from build123d import *

# Parameters (mm, degrees)
PAD018_DEPTH            = 12.35
PAD019_DEPTH            = 4.17
SKETCH036_R             = 1.5
POCKET011_DEPTH         = 5
FILLET014_R             = 0.3
BODY008_PLACEMENT_ANGLE = 180


with BuildPart() as part:
    # Sketch034 → Pad018 (new body)
    with BuildSketch(Plane.XY):
        Polygon((0, 23.8), (22.6, 23.8), (22.6, 19.97), (27.78, 19.97), (27.78, 17.33), (22.6, 17.33), (22.6, 0), (0, 0), (0, 17.33), (-5.18, 17.33), (-5.18, 19.97), (0, 19.97), align=None)
    extrude(amount=PAD018_DEPTH)

    # Sketch035 (on Face4 of Pad018) → Pad019 (join)
    with BuildSketch(Plane(origin=(0, 23.8, 0), x_dir=(-1, 0, 0), z_dir=(0, 1, 0))):
        with BuildLine():
            ThreePointArc((-10.895586, 8.809617), (-22.55, 6.175), (-10.895586, 3.540383))
            ThreePointArc((-10.895586, 3.540383), (-7.605, 6.175), (-10.895586, 8.809617))
        make_face()
    extrude(amount=PAD019_DEPTH)

    # Sketch036 (on Face10 of Pad019) → Pocket011 (cut)
    with BuildSketch(Plane(origin=(0, 19.97, 0), x_dir=(-1, 0, 0), z_dir=(0, 1, 0))):
        with Locations((-25.73, 6.175)):
            Circle(SKETCH036_R)
        with Locations((3.13, 6.175)):
            Circle(SKETCH036_R)
    extrude(amount=-POCKET011_DEPTH, mode=Mode.SUBTRACT)

    # Fillet014
    fillet014_edges = [part.edges().sort_by_distance(p)[0] for p in [
        (22.55, 27.97, 6.175),
        (7.605, 27.97, 6.175),
    ]]
    fillet(fillet014_edges, radius=FILLET014_R)


with BuildPart() as part_1:
    # Body008 placement: moved
    add(part.part.moved(Location((215.339996, 126.400008, -13.43))).rotate(Axis((215.339996, 126.400008, -13.43), (0, 1, 0)), BODY008_PLACEMENT_ANGLE))


solid = part_1.part
The model under review builds one solid part; all positions refer to its coordinate system, in mm. A direction names the side the tool comes from. Give positions to 0.01 mm unless a question says otherwise; leave off trailing zeros. Order: outer loops, then holes, each group sorted by start corner. A loop starts at its lowest first (then second) coordinate and runs counter-clockwise, first axis right, second up. Notation, with made-up numbers: M 73.25,35 L 119.25,35 A13 ccw 119.25,49 Z; hole C 72.5,65.25 d7. An arc over 180 degrees is marked long. One line per question, with ' | ' between items. Start each with the question number.
1) Clearance check with flat-ended pins moving along their axes: P1, Ø1.9, axis at y = 147.5, z = -21, coming from the +X side; P2, Ø1, axis at x = 212.5, z = -22.5, coming from the +Y side; P3, Ø2.5, axis at x = 189.61, z = -19.6, coming from the +Y side; P4, Ø1.6, axis at x = 216.5, z = -22.5, coming from the -Y side. State where each tip first meets the part, or that it passes through.
2) Mouldability with a two-part tool opening along Z and no side actions: class faces 1 (the face through (216.8, 146.37, -19.5)), 2 (the face through (219.9, 145.07, -20.06)), 3 (the face through (207.734, 152.108, -19.537)) as pulls with the +Z half, pulls with the -Z half, needs draft (parallel to the pull), parting line crosses it, or undercut.
3) Consider section C-C, the plane y = 133.25. Give the boundary of the cut face in (x, z), then the cut area to 3 significant figures.
4) Consider section A-A, the plane y = 145. Give the boundary of the cut face in (x, z) (3 decimals).
5) Consider section B-B, the plane z = -19. State how many separate pieces and enclosed holes the cut face has, then the cut area to 3 significant figures.
6) Wall thickness on L1, parallel to Y at x = 190, z = -15.25; L2, parallel to X at y = 132.5, z = -14; L3, parallel to Y at x = 203, z = -24.25: over which ranges is each line inside the solid? List them lowest first. Write a range as from..to.
7) For faces 4 (the face through (191.3, 146.37, -19.5)), 5 (the face through (192.794, 152.108, -19.836)), 6 (the face through (215.34, 148, -20)), 7 (the face through (215.34, 135, -20)), 8 (the face through (191.3, 143.73, -19.5)), list the 3-axis set-ups (+Z, -Z, +X, -X, +Y, -Y) from which the entire face can be reached by the end or side of a thin tool; tool diameter is ignored.
8) Consider section D-D, the plane x = 211. Give the boundary of the cut face in (y, z).
Found:
1) P1: stops at x = 215.34 | P2: stops at y = 150.2 | P3: passes through | P4: stops at y = 143.73
2) face 1: needs draft | face 2: undercut | face 3: parting line crosses it
3) outline: M 192.74,-25.78 L 215.34,-25.78 L 215.34,-13.43 L 192.74,-13.43 Z | area: 279 mm²
4) outline: M 187.56,-25.78 L 220.52,-25.78 L 220.52,-13.43 L 187.56,-13.43 Z; hole C 189.61,-19.605 d3; hole C 218.47,-19.605 d3
5) separate pieces: 3 | enclosed holes: 0 | area: 613 mm²
6) L1: y = 143.73..146.37 | L2: x = 192.74..215.34 | L3: y = 126.4..150.2
7) face 4: +Z, -Z, -X, +Y | face 5: +Y | face 6: +Z, -Z, +X, +Y | face 7: +Z, -Z, +X, -Y | face 8: +Z, -Z, -X, -Y
8) outline: M 126.4,-25.78 L 150.2,-25.78 L 150.2,-13.43 L 126.4,-13.43 Z
